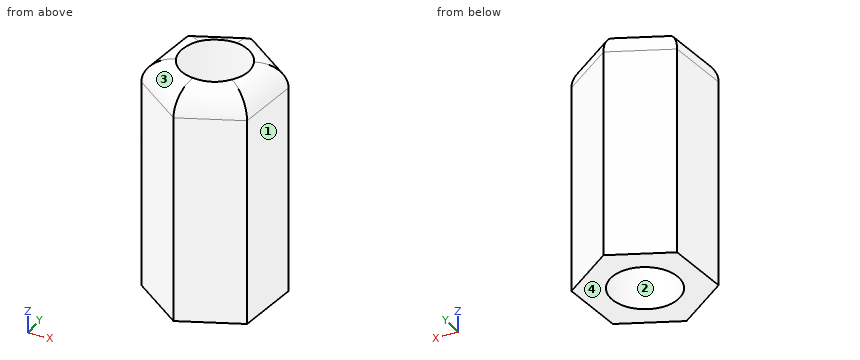
```python
from build123d import *

# Parameters (mm, degrees)
F0_R         = 4.05
F1_DEPTH     = 28
F2_T1_DEPTH  = 22.6428048889
F2_T3_DEPTH  = 22.6428048889
F2_T5_DEPTH  = 22.6428048889
F2_T7_DEPTH  = 22.6428048889
F2_T9_DEPTH  = 22.6428048889
F2_T11_DEPTH = 22.6428048889


# Not quite as in the source:
# - a fillet or chamfer that OpenCascade refuses, or shapes differently, is made with other operations: its cross-section is extruded or revolved along the edge and cut away or added


with BuildPart() as f1:
    # F0 (on Top) → F1 (new body)
    with BuildSketch(Plane.XY):
        Polygon((6.1779160549, -4.4995355079), (6.9856700826, 3.1004644921), (0.8077540276, 7.6), (-6.1779160549, 4.4995355079), (-6.9856700826, -3.1004644921), (-0.8077540276, -7.6), align=None)
        Circle(F0_R, mode=Mode.SUBTRACT)
    extrude(amount=F1_DEPTH)

    # F2: fillet of radius 3 on 6 edges, made by hand

    # F2_s2 → F2_t1 (cut)
    with BuildSketch(Plane(origin=(-10.3479787197, -4.5927649325, 0), x_dir=(0, 0, 1), z_dir=(0.9140191571, 0.4056710249, 0))):
        with BuildLine():
            ThreePointArc((25, 6.6188631899), (27.1213203436, 5.7401835335), (28, 3.6188631899))
            Line((28, 3.6188631899), (28, 6.6188631899))
            Line((28, 6.6188631899), (25, 6.6188631899))
        make_face()
    extrude(amount=F2_T1_DEPTH, mode=Mode.SUBTRACT)

    # F2_s4 → F2_t3 (cut)
    with BuildSketch(Plane(origin=(-9.151440465, 6.6652299829, 0), x_dir=(0, 0, 1), z_dir=(0.8083309917, -0.5887282972, 0))):
        with BuildLine():
            ThreePointArc((25, 6.6188631899), (27.1213203436, 5.7401835335), (28, 3.6188631899))
            Line((28, 3.6188631899), (28, 6.6188631899))
            Line((28, 6.6188631899), (25, 6.6188631899))
        make_face()
    extrude(amount=F2_T3_DEPTH, mode=Mode.SUBTRACT)

    # F2_s6 → F2_t5 (cut)
    with BuildSketch(Plane(origin=(1.1965382547, 11.2579949153, 0), x_dir=(0, 0, 1), z_dir=(-0.1056881655, -0.994399322, 0))):
        with BuildLine():
            ThreePointArc((25, 6.6188631899), (27.1213203436, 5.7401835335), (28, 3.6188631899))
            Line((28, 3.6188631899), (28, 6.6188631899))
            Line((28, 6.6188631899), (25, 6.6188631899))
        make_face()
    extrude(amount=F2_T5_DEPTH, mode=Mode.SUBTRACT)

    # F2_s8 → F2_t7 (cut)
    with BuildSketch(Plane(origin=(10.3479787197, 4.5927649325, 0), x_dir=(0, 0, 1), z_dir=(-0.9140191571, -0.4056710249, 0))):
        with BuildLine():
            ThreePointArc((25, 6.6188631899), (27.1213203436, 5.7401835335), (28, 3.6188631899))
            Line((28, 3.6188631899), (28, 6.6188631899))
            Line((28, 6.6188631899), (25, 6.6188631899))
        make_face()
    extrude(amount=F2_T7_DEPTH, mode=Mode.SUBTRACT)

    # F2_s10 → F2_t9 (cut)
    with BuildSketch(Plane(origin=(9.151440465, -6.6652299829, 0), x_dir=(0, 0, 1), z_dir=(-0.8083309917, 0.5887282972, 0))):
        with BuildLine():
            ThreePointArc((25, 6.6188631899), (27.1213203436, 5.7401835335), (28, 3.6188631899))
            Line((28, 3.6188631899), (28, 6.6188631899))
            Line((28, 6.6188631899), (25, 6.6188631899))
        make_face()
    extrude(amount=F2_T9_DEPTH, mode=Mode.SUBTRACT)

    # F2_s12 → F2_t11 (cut)
    with BuildSketch(Plane(origin=(-1.1965382547, -11.2579949153, 0), x_dir=(0, 0, 1), z_dir=(0.1056881655, 0.994399322, 0))):
        with BuildLine():
            ThreePointArc((25, 6.6188631899), (27.1213203436, 5.7401835335), (28, 3.6188631899))
            Line((28, 3.6188631899), (28, 6.6188631899))
            Line((28, 6.6188631899), (25, 6.6188631899))
        make_face()
    extrude(amount=F2_T11_DEPTH, mode=Mode.SUBTRACT)


solid = f1.part
```
CAD build for the part. Positions are in the model's coordinates, mm. Face numbers are marked on the shaded views. Round coordinates to 2 decimals unless told otherwise and drop trailing zeros. Write each loop counter-clockwise with the first axis right and the second up, starting at its lowest first coordinate (ties: lowest second). Pieces come first, ordered by that corner, then holes. Notation, with made-up numbers: (42, 33) - (50, 33) arc R12 ccw to (50, 41) - close; hole circle Ø3 at (65, -15.5). An arc over 180 degrees is marked (long way). Return JSON: item names as keys, results as strings. Group by question number.
Item 1: Probe probe 1 along X at (y, z) = (2.75, 14.5); probe 2 along X at (y, z) = (0, 17.5); probe 3 along Y at (x, z) = (2.5, 2). List the from-to ranges inside material, lowest first.
Item 2: Mould opens along X. For the marked faces 1, 2, 3 and 4 say: +X half, -X half, draft (parallel to the pull), parting line (faces both ways), or undercut.
Item 3: Band-saw the part on B-B on z = 25.5. List the corners of the cut face in (x, y), plus the area to 3 significant figures.
Item 4: Flat gauge pins, fed straight in: pin 1 Ø5 at (x, y) = (0, 0) entering from -Z; pin 2 Ø4 at (x, y) = (3.5, 6) entering from +Z; pin 3 Ø1.5 at (x, z) = (4, 16.5) entering from -Y; pin 4 Ø6 at (x, z) = (-3, 22) entering from +Y. Where does each tip first touch, or does it go through?
Item 5: Band-saw the part on A-A on z = 4. List the corners of the cut face in (x, y).
Resolved:
{
 "1": {"probe 1": "x = -6.36 to -2.97, 2.97 to 6.95", "probe 2": "x = -6.66 to -4.05, 4.05 to 6.66", "probe 3": "y = -6.13 to -3.19, 3.19 to 6.37"},
 "2": {"face 1": "+X half", "face 2": "undercut", "face 3": "-X half", "face 4": "draft"},
 "3": {"outline": "(-6.94, -3.08) - (-0.8, -7.55) - (6.14, -4.47) - (6.94, 3.08) - (0.8, 7.55) - (-6.14, 4.47) - close; hole circle Ø8.1 at (0, 0)", "area": "98.3 mm²"},
 "4": {"pin 1": "passes through", "pin 2": "stops at z = 27.71", "pin 3": "stops at y = -5.8", "pin 4": "stops at y = 7.24"},
 "5": {"outline": "(-6.99, -3.1) - (-0.81, -7.6) - (6.18, -4.5) - (6.99, 3.1) - (0.81, 7.6) - (-6.18, 4.5) - close; hole circle Ø8.1 at (0, 0)"}
}
